```python
from build123d import *

# Parameters (mm, degrees)
BOSS_EXTRUDE1_DEPTH = 1
FILLET1_R           = 0.5


with BuildPart() as part:
    # Sketch1 → Boss-Extrude1 (new body)
    with BuildSketch(Plane(origin=(0, 0, 0), x_dir=(1, 0, 0), z_dir=(0, 1, 0))):
        with BuildLine():
            Line((0, 2.5), (4.026491886, 2.5))
            Line((4.026491886, 2.5), (4.026491886, 6.055714934))
            Line((4.026491886, 6.055714934), (-2.5, 6.055714934))
            ThreePointArc((-2.5, 6.055714934), (-8.555714934, 0), (-2.5, -6.055714934))
            Line((-2.5, -6.055714934), (4.026491886, -6.055714934))
            Line((4.026491886, -6.055714934), (4.026491886, -2.5))
            Line((4.026491886, -2.5), (0, -2.5))
            ThreePointArc((0, -2.5), (-2.5, 0), (0, 2.5))
        make_face()
    extrude(amount=BOSS_EXTRUDE1_DEPTH)

    # Fillet1
    fillet1_edges = [part.edges().sort_by_distance(p)[0] for p in [
        (0.763245943, 0, -6.055714934),
        (0.763245943, 0, 6.055714934),
        (0.763245943, 1, -6.055714934),
        (0.763245943, 1, 6.055714934),
        (-8.555714934, 0, 0),
        (-8.555714934, 1, 0),
    ]]
    fillet(fillet1_edges, radius=FILLET1_R - 0.0001)  # a hair under: the kernel refuses the full size


solid = part.part
```
Design review of the part built by this model. Coordinates are the model's own, in mm. A direction names the side the tool comes from. Give positions to 0.01 mm unless a question says otherwise; leave off trailing zeros. Order: outer loops, then holes, each group sorted by start corner. A loop starts at its lowest first (then second) coordinate and runs counter-clockwise, first axis right, second up. Notation, with made-up numbers: (9, -1.5) -> (30, -1.5) arc R34 ccw to (30, 31.5) -> close; hole circle Ø1 at (50.5, -28). An arc over 180 degrees is marked (long way). Write item = value, one per line. Start each with the question number.
(1) For faces 1 (the face through (4.026, 0.5, -4.3)), 2 (the face through (2, 0.5, 2.5)), list the 3-axis set-ups (+Z, -Z, +X, -X, +Y, -Y) from which the entire face can be reached by the end or side of a thin tool; tool diameter is ignored.
(2) To check wall thickness, follow line 1 along Z through (x, y) = (3, 0.7); line 2 along X through (y, z) = (0.45, 0); line 3 along X through (y, z) = (0.9, 3.5). State the ranges of each line that lie inside material, in increasing order.
(3) Mouldability with a two-part tool opening along Z and no side actions: class faces 3 (the face through (2, 0.5, -2.5)), 4 (the face through (-3, 0, 0)), 5 (the face through (-2.5, 0.5, 0.1)) as +Z half, -Z half, draft (parallel to the pull), parting line (faces both ways), or undercut.
(4) For pin 1 (1.5 mm diameter, centred on x = -5, z = 4.5, fed in from -Y), flat-tipped, find the tip position at first contact; note if it passes through.
(5) We need section B-B on y = 0.2. Write out the cut boundary in (x, z), plus the area to 3 significant figures.
Numbers:
q1.face_1 = +Z, -Z, +X, +Y, -Y
q1.face_2 = +X, +Y, -Y
q2.line_1 = -6.01 to -2.5, 2.5 to 6.01
q2.line_2 = -8.55 to -2.5
q2.line_3 = -7.19 to 4.03
q3.face_3 = undercut
q3.face_4 = draft
q3.face_5 = undercut
q4.pin_1 = 0
q5.outline = (-2.5, -5.96) -> (4.03, -5.96) -> (4.03, -2.5) -> (0, -2.5) arc R2.5 cw to (0, 2.5) -> (4.03, 2.5) -> (4.03, 5.96) -> (-2.5, 5.96) arc R5.96 ccw to start
q5.area = 104 mm^2
